Job drawing, mm, ordinate dimensions from the low corner. One solid piece. Give positions to 0.01 mm unless a question says otherwise; leave off trailing zeros. Write each loop counter-clockwise with the first axis right and the second up, starting at its lowest first coordinate (ties: lowest second). Pieces come first, ordered by that corner, then holes. Notation, with made-up numbers: (7, 72) -> (17, 72) arc R20 ccw to (17, 98) -> close; hole circle Ø2 at (57, 44). An arc over 180 degrees is marked (long way). Put each result on its own line as item: value. Start each with the question number.
Item 1: Slice it at A-A, the plane x = 16. List the corners of the cut face in (y, z).
Item 2: Flat gauge pin, fed straight in: pin 1 Ø2 at (x, z) = (5.5, 6) entering from +Y. Where does the tip first touch, or does it go through?
Item 3: Slice it at C-C, the plane z = 2.5. List the corners of the cut face in (x, y), plus the area to 3 significant figures.
Item 4: Drill centre lines: line 1 along Y through (x, z) = (21.5, 3.75); line 2 along X through (y, z) = (189, 1.25); line 3 along Y through (x, z) = (30.5, 9.25). Where is each one in solid material? Low to high.
Item 5: Slice it at B-B, the plane y = 176. List the corners of the cut face in (x, z).
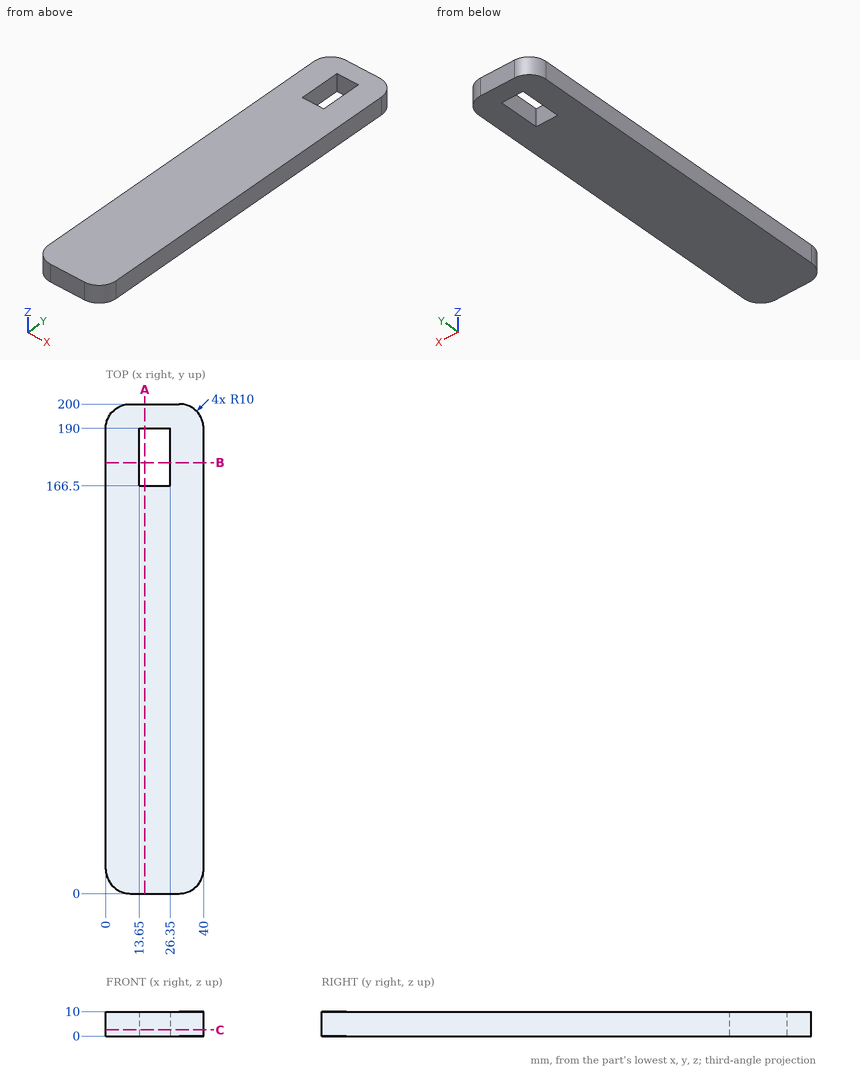
Values follow:
1. outline: (0, 0) -> (166.5, 0) -> (166.5, 10) -> (0, 10) -> close; (190, 0) -> (200, 0) -> (200, 10) -> (190, 10) -> close
2. pin 1: y = 199.37
3. outline: (0, 10) arc R10 ccw to (10, 0) -> (30, 0) arc R10 ccw to (40, 10) -> (40, 190) arc R10 ccw to (30, 200) -> (10, 200) arc R10 ccw to (0, 190) -> close; hole (13.65, 166.5) -> (26.35, 166.5) -> (26.35, 190) -> (13.65, 190) -> close
3. area: 7,620 mm2
4. line 1: 0 to 166.5, 190 to 200
4. line 2: 0 to 13.65, 26.35 to 40
4. line 3: 0.01 to 199.99
5. outline: (0, 0) -> (13.65, 0) -> (13.65, 10) -> (0, 10) -> close; (26.35, 0) -> (40, 0) -> (40, 10) -> (26.35, 10) -> close
